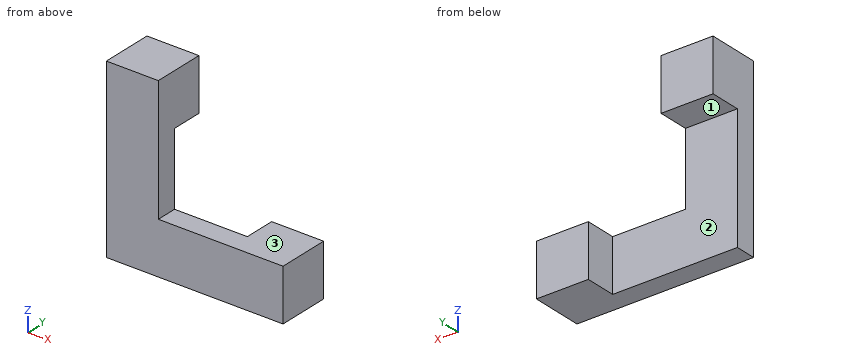
```python
from build123d import *

# Parameters (mm, degrees)
BOSS_EXTRUDE1_DEPTH = 2
SKETCH2_W           = 5
SKETCH2_H           = 5
BOSS_EXTRUDE2_DEPTH = 5


with BuildPart() as part:
    # Sketch1 → Boss-Extrude1 (new body)
    with BuildSketch(Plane(origin=(0, 0, 0), x_dir=(1, 0, 0), z_dir=(0, 1, 0))):
        Polygon((0, 0), (0, 7), (7, 7), (7, 12), (-5, 12), (-5, 0), align=None)
    extrude(amount=BOSS_EXTRUDE1_DEPTH)

    # Sketch2 → Boss-Extrude2 (add)
    with BuildSketch(Plane.XZ):
        with Locations((-2.5, 2.5)):
            Rectangle(SKETCH2_W, SKETCH2_H)
        with Locations((9.5, -9.5)):
            Rectangle(SKETCH2_W, SKETCH2_H)
    extrude(amount=-BOSS_EXTRUDE2_DEPTH)


solid = part.part
```
Source: CAD feature listing. Evaluate the final solid. Frame: model axes, mm. Face numbers are marked on the shaded views. A direction names the side the tool comes from. Give positions to 0.01 mm unless a question says otherwise; leave off trailing zeros. Loops run counter-clockwise (first coordinate to the right, second up) from the corner with the lowest first, then second, coordinate; pieces in that order, holes last. Notation, with made-up numbers: (30.25, -22.5) -> (49.25, -22.5) arc R17 cw to (49.25, 0.5) -> close; hole circle Ø6 at (-31, -21.75). An arc over 180 degrees is marked (long way). Put each result on its own line as item: value. Start each with the question number.
1) Cut plane C-C (z = -3.5). Return loops of the section in (x, y), then the cut area to 3 significant figures.
2) Material intervals for probe 1 along Y at (x, z) = (-2.25, -4); probe 2 along X at (y, z) = (1.6, -0.25); probe 3 along Z at (x, y) = (8.5, 3.55), sorted ascending.
3) Cut plane B-B (x = -1). Return loops of the section in (y, z).
4) Cut plane D-D (y = 1.05). Return loops of the section in (x, z), then the cut area to 3 significant figures.
5) Reachability of the marked faces 1, 2 and 3 from +Z, -Z, +X, -X, +Y, -Y: full face, straight path, thin tool, end or side. Return the list, or none.
6) Cut plane A-A (y = 2.9). Return loops of the section in (x, z), then the cut area to 3 significant figures.
7) Contact query for flat-ended pins moving along their axis: P1, Ø1.5, axis at x = 10, z = -4.5, coming from the +Y side; P2, Ø3, axis at x = 2, y = 2.5, coming from the -Z side; P3, Ø2, axis at y = 4, z = 3, coming from the +X side; P4, Ø0.9, axis at y = 4, z = -9, coming from the -X side. Output: stop coordinate, or through.
Results are:
1. outline: (-5, 0) -> (0, 0) -> (0, 2) -> (-5, 2) -> close
1. area: 10.0 mm2
2. probe 1: y = 0 to 2
2. probe 2: x = -5 to 0
2. probe 3: z = -12 to -7
3. outline: (0, -12) -> (2, -12) -> (2, 0) -> (5, 0) -> (5, 5) -> (0, 5) -> close
4. outline: (-5, -12) -> (12, -12) -> (12, -7) -> (0, -7) -> (0, 5) -> (-5, 5) -> close
4. area: 145 mm2
5. face 1: -Z, +X, -X, +Y
5. face 2: -Z, -X, +Y
5. face 3: +Z, +X, +Y, -Y
6. outline: (-5, 0) -> (0, 0) -> (0, 5) -> (-5, 5) -> close; (7, -12) -> (12, -12) -> (12, -7) -> (7, -7) -> close
6. area: 50.0 mm2
7. P1: passes through
7. P2: stops at z = -12
7. P3: stops at x = 0
7. P4: stops at x = 7
